Verification items for the finished model (mm, model axes). Give positions to 0.01 mm unless a question says otherwise; leave off trailing zeros. Write each question's results on one line, items separated by ' | '. Start each with the question number.
```python
from build123d import *

# Parameters (mm, degrees)
SKIZZE1_W                       = 12
SKIZZE1_H                       = 4
AUFSATZ_LINEAR_AUSTRAGEN1_DEPTH = 580
SKIZZE2_R                       = 3
SCHNITT_LINEAR_AUSTRAGEN1_DEPTH = 581.137914638


with BuildPart() as part:
    # Skizze1 → Aufsatz-Linear austragen1 (new body)
    with BuildSketch(Plane.XY):
        with Locations((6, 2)):
            Rectangle(SKIZZE1_W, SKIZZE1_H)
    extrude(amount=AUFSATZ_LINEAR_AUSTRAGEN1_DEPTH)

    # Skizze2 → Schnitt-Linear austragen1 (cut, through all)
    with BuildSketch(Plane(origin=(0, 4, 0), x_dir=(1, 0, 0), z_dir=(0, 1, 0))):
        with Locations(Location((6, -10, 0), (0, 0, 270))):
            Circle(SKIZZE2_R)
        with Locations(Location((6, -20, 0), (0, 0, 270))):
            Circle(SKIZZE2_R)
        with Locations(Location((6, -30, 0), (0, 0, 270))):
            Circle(SKIZZE2_R)
        with Locations(Location((6, -40, 0), (0, 0, 270))):
            Circle(SKIZZE2_R)
        with Locations(Location((6, -50, 0), (0, 0, 270))):
            Circle(SKIZZE2_R)
        with Locations(Location((6, -60, 0), (0, 0, 270))):
            Circle(SKIZZE2_R)
        with Locations(Location((6, -70, 0), (0, 0, 270))):
            Circle(SKIZZE2_R)
        with Locations(Location((6, -80, 0), (0, 0, 270))):
            Circle(SKIZZE2_R)
        with Locations(Location((6, -90, 0), (0, 0, 270))):
            Circle(SKIZZE2_R)
        with Locations(Location((6, -100, 0), (0, 0, 270))):
            Circle(SKIZZE2_R)
        with Locations(Location((6, -110, 0), (0, 0, 270))):
            Circle(SKIZZE2_R)
        with Locations(Location((6, -120, 0), (0, 0, 270))):
            Circle(SKIZZE2_R)
        with Locations(Location((6, -130, 0), (0, 0, 270))):
            Circle(SKIZZE2_R)
        with Locations(Location((6, -450, 0), (0, 0, 90))):
            Circle(SKIZZE2_R)
        with Locations(Location((6, -460, 0), (0, 0, 90))):
            Circle(SKIZZE2_R)
        with Locations(Location((6, -470, 0), (0, 0, 90))):
            Circle(SKIZZE2_R)
        with Locations(Location((6, -480, 0), (0, 0, 90))):
            Circle(SKIZZE2_R)
        with Locations(Location((6, -490, 0), (0, 0, 90))):
            Circle(SKIZZE2_R)
        with Locations(Location((6, -500, 0), (0, 0, 90))):
            Circle(SKIZZE2_R)
        with Locations(Location((6, -510, 0), (0, 0, 90))):
            Circle(SKIZZE2_R)
        with Locations(Location((6, -520, 0), (0, 0, 90))):
            Circle(SKIZZE2_R)
        with Locations(Location((6, -530, 0), (0, 0, 90))):
            Circle(SKIZZE2_R)
        with Locations(Location((6, -540, 0), (0, 0, 90))):
            Circle(SKIZZE2_R)
        with Locations(Location((6, -550, 0), (0, 0, 90))):
            Circle(SKIZZE2_R)
        with Locations(Location((6, -560, 0), (0, 0, 90))):
            Circle(SKIZZE2_R)
        with Locations(Location((6, -570, 0), (0, 0, 90))):
            Circle(SKIZZE2_R)
    extrude(amount=-SCHNITT_LINEAR_AUSTRAGEN1_DEPTH, mode=Mode.SUBTRACT)


solid = part.part
```
1. Depth check by flat-ended pin: pin 1 Ø7 at (x, z) = (6, 510) entering from +Y. Enter the tip coordinate at first touch or a pass-through.
2. Section check A-A, the plane y = 2.9. State how many separate pieces and enclosed holes the cut face has, plus the area to 3 significant figures.
3. Thickness scan on probe 1 along X at (y, z) = (1.75, 530); probe 2 along X at (y, z) = (1.65, 111). Record the ranges inside material, lowest first.
Filled sheet:
1) pin 1: y = 4
2) separate pieces: 1 | enclosed holes: 26 | area: 6,220 mm2
3) probe 1: 0 to 3, 9 to 12 | probe 2: 0 to 3.17, 8.83 to 12
